Autodesk Inventor part; units mm, degrees
ref_plane "YZ Plane" through (0, 0, 0) normal (1, 0, 0) x (0, 1, 0)
ref_plane "XZ Plane" through (0, 0, 0) normal (0, 1, 0) x (-1, 0, 0)
ref_plane "XY Plane" through (0, 0, 0) normal (0, 0, 1) x (1, 0, 0)
sketch "Sketch1" plane through (0, 0, 0) normal (0, 0, 1) x (1, 0, 0)
  line L0 (0, 0) -> (43.38, 0)
  line L1 (43.38, 0) -> (43.38, 18.44)
  line L2 (43.38, 18.44) -> (0, 18.44)
  line L3 (0, 18.44) -> (0, 0)
  circle A0 centre (1.5, 16.94) radius 0.85
  circle A1 centre (1.5, 1.5) radius 0.85
  circle A2 centre (41.88, 16.94) radius 0.85
  circle A3 centre (41.88, 1.5) radius 0.85
  dimension "d0" = 43.38
  dimension "d1" = 18.44
  dimension "d2" = 1.7
  dimension "d3" = 1.5
  dimension "d4" = 1.5
  dimension "d5" = 1.5
  dimension "d6" = 1.5
extrude "Extrusion1" add sketch "Sketch1" along normal blind 1.53
sketch "Sketch2" plane through (0, 0, 1.53) normal (0, 0, 1) x (1, 0, 0)
  line L0 (23.1338, 9.22) -> (27.73, 13.8162)
  line L1 (27.73, 13.8162) -> (32.3262, 9.22)
  line L2 (32.3262, 9.22) -> (27.73, 4.6238)
  line L3 (27.73, 4.6238) -> (23.1338, 9.22)
  line L4 (0, 0) -> (43.38, 0)
  line L5 (0, 18.44) -> (0, 0)
  line L6 (43.38, 0) -> (43.38, 18.44)
  line L7 (35.86, 5.42) -> (45.11, 5.42)
  line L8 (45.11, 5.42) -> (45.11, 13.02)
  line L9 (45.11, 13.02) -> (35.86, 13.02)
  line L10 (35.86, 13.02) -> (35.86, 5.42)
  point P0 (0, 9.22)
  point P1 (45.11, 9.22)
  dimension "d9" = 45
  dimension "d10" = 6.5
  dimension "d11" = 15.65
  dimension "d12" = 9.25
  dimension "d13" = 7.6
  dimension "d14" = 1.73
extrude "Extrusion2" add sketch "Sketch2" along normal blind 3.75 contours L7 L10 L9 L6 | L6 L9 L8 L7
extrude "Extrusion3" add sketch "Sketch2" along normal blind 0.8 contours L0 L1 L2 L3
fillet "Fillet1" radius 0.5 2 edges at (40.485, 5.42, 5.28) (40.485, 13.02, 5.28)
properties part number "MICROCONTROLLER"
Could you check a few things on this model? Use its own coordinates, in mm. A direction names the side the tool comes from. Round coordinates to 2 decimals unless told otherwise and drop trailing zeros. Loops run counter-clockwise (first coordinate to the right, second up) from the corner with the lowest first, then second, coordinate; pieces in that order, holes last. Notation, with made-up numbers: M 64,-6.5 L 71,-6.5 A20 cw 71,30.5 Z; hole C 33,36.25 d6. An arc over 180 degrees is marked long. Put each result on its own line as item: value.
Q1. Imagine slicing it at B-B (y = 1.5). Write out the boundary of the cut face in (x, z), then the cut area to 3 significant figures.
Check result:
outline: M 0,0 L 0.65,0 L 0.65,1.53 L 0,1.53 Z; M 2.35,0 L 41.03,0 L 41.03,1.53 L 2.35,1.53 Z; M 42.73,0 L 43.38,0 L 43.38,1.53 L 42.73,1.53 Z
area: 61.2 mm2
Q2. I need wall thicknesses on probe 1 along Y at (x, z) = (1.5, 0.5); probe 2 along Z at (x, y) = (3.5, 8.75); probe 3 along Z at (x, y) = (25.5, 10.5). Which ranges of each line are inside material? Lowest first, please.
Check result:
probe 1: 0 to 0.65, 2.35 to 16.09, 17.79 to 18.44
probe 2: 0 to 1.53
probe 3: 0 to 2.33
Q3. On a 3-axis mill with a long thin cutter (end or side, diameter ignored), from which of +Z, -Z, +X, -X, +Y, -Y can I reach the whole of each face in a straight line? I mean faces 1 (the face through (44, 9, 1.53)), 2 (the face through (28, 9, 2.33)), 3 (the face through (40, 5.42, 3)). Say none if no direction works.
Check result:
face 1: -Z, +X, +Y, -Y
face 2: +Z, -X, +Y, -Y
face 3: +Z, +X, -Y
Q4. Imagine slicing it at D-D (x = 1.5). Write out the boundary of the cut face in (y, z), then the cut area to 3 significant figures.
Check result:
outline: M 0,0 L 0.65,0 L 0.65,1.53 L 0,1.53 Z; M 2.35,0 L 16.09,0 L 16.09,1.53 L 2.35,1.53 Z; M 17.79,0 L 18.44,0 L 18.44,1.53 L 17.79,1.53 Z
area: 23.0 mm2
Q5. Imagine slicing it at C-C (z = 0.8). Write out the boundary of the cut face in (x, y), then the cut area to 3 significant figures.
Check result:
outline: M 0,0 L 43.38,0 L 43.38,18.44 L 0,18.44 Z; hole C 1.5,1.5 d1.7; hole C 1.5,16.94 d1.7; hole C 41.88,1.5 d1.7; hole C 41.88,16.94 d1.7
area: 791 mm2
Q6. Imagine slicing it at A-A (x = 41.88). Write out the boundary of the cut face in (y, z).
Check result:
outline: M 0,0 L 0.65,0 L 0.65,1.53 L 0,1.53 Z; M 2.35,0 L 16.09,0 L 16.09,1.53 L 13.02,1.53 L 13.02,4.78 A0.5 ccw 12.52,5.28 L 5.92,5.28 A0.5 ccw 5.42,4.78 L 5.42,1.53 L 2.35,1.53 Z; M 17.79,0 L 18.44,0 L 18.44,1.53 L 17.79,1.53 Z
Q7. For pin 1 (2.5 mm diameter, centred on x = 41.88, y = 1.5, fed in from +Z); pin 2 (3 mm diameter, centred on y = 9, z = 3.5, fed in from -X); pin 3 (5.5 mm diameter, centred on x = 22, y = 8.5, fed in from +Z); pin 4 (1 mm diameter, centred on y = 2.5, z = 4, fed in from -X), each with a flat end and sliding along its axis, tell me the tip position at first contact or that it passes through.
Check result:
pin 1: z = 1.53
pin 2: x = 23.13
pin 3: z = 2.33
pin 4: through
Q8. Thinking about a two-plate mould opening in X: for faces 4 (the face through (29.996, 11.55, 1.924)), 5 (the face through (41, 13.02, 3)), 6 (the face through (43.38, 9, 1)), 7 (the face through (0, 9, 1)), which applies, released by +X, released by -X, zero draft, split by the parting line, or undercut?
Check result:
face 4: undercut
face 5: zero draft
face 6: released by +X
face 7: released by -X
